Here's how the part is built. I have some questions about the finished solid (model axes, mm). A direction names the side the tool comes from. Give positions to 0.01 mm unless a question says otherwise; leave off trailing zeros. Order: outer loops, then holes, each group sorted by start corner. A loop starts at its lowest first (then second) coordinate and runs counter-clockwise, first axis right, second up. Notation, with made-up numbers: (-16.5, -21) -> (26.5, -21) arc R23 ccw to (26.5, -13) -> close; hole circle Ø6 at (55.25, -20). An arc over 180 degrees is marked (long way). Write each question's results on one line, items separated by ' | '. Start each with the question number.
Q1. Imagine slicing it at C-C, the plane x = -15. Please give me the cut outline in (y, z), then the cut area to 3 significant figures.
Q2. I need wall thicknesses on line 1 along Y through (x, z) = (6, 35.5); line 2 along X through (y, z) = (2, -22); line 3 along X through (y, z) = (1.5, 29). Which ranges of each line are inside material? Lowest first, please. Write a range as [from, to].
Q3. Imagine slicing it at B-B, the plane z = 15.5. Please give me the cut outline in (x, y).
Q4. For faces 1 (the face through (-25, 4.064, -25)), 2 (the face through (-1, 0, 1)), which set-ups out of +Z, -Z, +X, -X, +Y, -Y let a thin tool reach every point of the face, with its end or its side?
Q5. Imagine slicing it at A-A, the plane y = 3. Please give me the cut outline in (x, z).
Q6. I'm going to push a flat-ended pin straight in: pin 1 (2 mm diameter, centred on x = 26.5, z = 9.5, fed in from +Y). Where does the tip first touch, or does it pass through?
Q7. Imagine slicing it at D-D, the plane z = -28.5. Please give me the cut outline in (x, y).
```python
from build123d import *

# Parameters (mm, degrees)
F0_W     = 76.2
F0_H     = 76.2
F1_DEPTH = 2.286
F3_DEPTH = 4.064


with BuildPart() as f1:
    # F0 (on Front) → F1 (new body)
    with BuildSketch(Plane.XZ):
        Rectangle(F0_W, F0_H)
    extrude(amount=F1_DEPTH)

    # F2 (on face) → F3 (join)
    with BuildSketch(Plane(origin=(0, 0, 0), x_dir=(-1, 0, 0), z_dir=(0, 1, 0))):
        with BuildLine():
            ThreePointArc((20.8367786429, -20.8367786429), (20.8367786429, -29.8170347639), (29.8170347639, -29.8170347639))
            Line((29.8170347639, -29.8170347639), (20.8367786429, -20.8367786429))
        make_face()
        with BuildLine():
            Line((-20.8367786429, -20.8367786429), (-29.8170347639, -29.8170347639))
            ThreePointArc((-29.8170347639, -29.8170347639), (-22.8968669079, -31.1935417349), (-18.9769067034, -25.3269067034))
            ThreePointArc((-18.9769067034, -25.3269067034), (-19.460271672, -22.8968669079), (-20.8367786429, -20.8367786429))
        make_face()
        with BuildLine():
            ThreePointArc((-20.8367786429, -20.8367786429), (-29.8170347639, -20.8367786429), (-29.8170347639, -29.8170347639))
            Line((-29.8170347639, -29.8170347639), (-20.8367786429, -20.8367786429))
        make_face()
        with BuildLine():
            Line((-20.8367786429, 20.8367786429), (-29.8170347639, 29.8170347639))
            ThreePointArc((-29.8170347639, 29.8170347639), (-29.8170347639, 20.8367786429), (-20.8367786429, 20.8367786429))
        make_face()
        with BuildLine():
            ThreePointArc((-18.9769067034, 25.3269067034), (-22.8968669079, 31.1935417349), (-29.8170347639, 29.8170347639))
            Line((-29.8170347639, 29.8170347639), (-20.8367786429, 20.8367786429))
            ThreePointArc((-20.8367786429, 20.8367786429), (-19.460271672, 22.8968669079), (-18.9769067034, 25.3269067034))
        make_face()
        with BuildLine():
            Line((20.8367786429, 20.8367786429), (29.8170347639, 29.8170347639))
            ThreePointArc((29.8170347639, 29.8170347639), (20.8367786429, 29.8170347639), (20.8367786429, 20.8367786429))
        make_face()
        with BuildLine():
            ThreePointArc((31.6769067034, 25.3269067034), (31.1935417349, 27.7569464989), (29.8170347639, 29.8170347639))
            Line((29.8170347639, 29.8170347639), (20.8367786429, 20.8367786429))
            ThreePointArc((20.8367786429, 20.8367786429), (27.7569464989, 19.460271672), (31.6769067034, 25.3269067034))
        make_face()
        with BuildLine():
            Line((20.8367786429, -20.8367786429), (29.8170347639, -29.8170347639))
            ThreePointArc((29.8170347639, -29.8170347639), (31.1935417349, -27.7569464989), (31.6769067034, -25.3269067034))
            ThreePointArc((31.6769067034, -25.3269067034), (27.7569464989, -19.460271672), (20.8367786429, -20.8367786429))
        make_face()
    extrude(amount=F3_DEPTH)


solid = f1.part
```
Geometry check:
1) outline: (-2.29, -38.1) -> (0, -38.1) -> (0, 38.1) -> (-2.29, 38.1) -> close | area: 174 mm²
2) line 1: [-2.29, 0] | line 2: [-30.74, -19.92], [19.92, 30.74] | line 3: [-30.51, -20.15], [20.15, 30.51]
3) outline: (-38.1, -2.29) -> (38.1, -2.29) -> (38.1, 0) -> (-38.1, 0) -> close
4) face 1: +Z, -Z, +X, -X, +Y | face 2: +Y
5) outline: circle Ø12.7 at (-25.33, -25.33); circle Ø12.7 at (-25.33, 25.33); circle Ø12.7 at (25.33, -25.33); circle Ø12.7 at (25.33, 25.33)
6) pin 1: y = 0
7) outline: (-38.1, -2.29) -> (38.1, -2.29) -> (38.1, 0) -> (30.83, 0) -> (30.83, 4.06) -> (19.83, 4.06) -> (19.83, 0) -> (-19.83, 0) -> (-19.83, 4.06) -> (-30.83, 4.06) -> (-30.83, 0) -> (-38.1, 0) -> close
